The model under review builds one solid part; all positions refer to its coordinate system, in mm. Face numbers are marked on the shaded views. A direction names the side the tool comes from. Coordinates: 2 decimals unless noted, no trailing zeros. Order: outer loops, then holes, each group sorted by start corner. A loop starts at its lowest first (then second) coordinate and runs counter-clockwise, first axis right, second up. Notation, with made-up numbers: (17, 66) - (74, 66) arc R20 ccw to (74, 101) - close; hole circle Ø3 at (-7.75, 13). An arc over 180 degrees is marked (long way). Answer in a Markdown table with one row per item.
Autodesk Inventor part; units mm, degrees
ref_plane "YZ Plane" through (0, 0, 0) normal (1, 0, 0) x (0, 1, 0)
ref_plane "XZ Plane" through (0, 0, 0) normal (0, 1, 0) x (-1, 0, 0)
ref_plane "XY Plane" through (0, 0, 0) normal (0, 0, 1) x (1, 0, 0)
sketch "スケッチ1" plane through (0, 0, 0) normal (1, 0, 0) x (0, 1, 0)
  line L0 (-6.5, 0) -> (6.5, 0)
  line L1 (0, 0) -> (0, 3.1754) construction
  line L2 (-6.2544, 3.1754) -> (-6.5, 2.75)
  line L3 (-6.5, 2.75) -> (-6.5, 0)
  line L4 (-6.2544, 3.1754) -> (6.2544, 3.1754)
  line L5 (6.2544, 3.1754) -> (6.5, 2.75)
  line L6 (6.5, 2.75) -> (6.5, 0)
  line L7 (-6.5, 1.5) -> (-12.2, 1.5)
  line L8 (-12.5, 1.2) -> (-12.5, 0)
  line L9 (-12.5, 0) -> (-6.5, 0)
  line L10 (-12.2, 1.5) -> (-12.5, 1.2)
  point P0 (6.5, 1.5)
  point P1 (-12.5, 1.5)
  dimension "d1" = 2.75
  dimension "d2" = 3.1754
  dimension "d3" = 30
  dimension "d4" = 13
  dimension "d18" = 6
  dimension "d19" = 3
  dimension "d22" = 0.3
  dimension "d23" = 0.3
revolve "回転1" add sketch "スケッチ1" angle 360 about axis through (0, -6.5, 0) along (0, 1, 0)
sketch "スケッチ2" plane through (0, 6.5, 0) normal (0, 1, 0) x (1, 0, 0)
  line L0 (0, -3.1754) -> (-2.75, -1.5877)
  line L1 (-2.75, -1.5877) -> (-2.75, 1.5877)
  line L2 (-2.75, 1.5877) -> (0, 3.1754)
  line L3 (0, 3.1754) -> (2.75, 1.5877)
  line L4 (2.75, 1.5877) -> (2.75, -1.5877)
  line L5 (2.75, -1.5877) -> (0, -3.1754)
  circle A0 centre (0, 0) radius 3.1754
  point P0 (0, 0)
  point P1 (0, 0)
  point P2 (0, 3.1754)
  point P3 (0, 3.1754)
  point P4 (2.75, -1.5877)
  point P5 (2.75, -1.5877)
extrude "押し出し1" cut sketch "スケッチ2" against normal through all contours A0 L0 | L5 A0 | A0 L1 | L4 A0 | A0 L2 | L3 A0
hole "穴1" at (0, 6.5, 0) direction (0, -1, 0) diameter 2.459 depth 3.3 tip angle 118 countersink diameter 3 countersink angle 90
thread "ねじ1"
equation "\"d2\" = 1.1547 * d1"
properties part number "BSL-313BE" material "アセタール樹脂、黒"
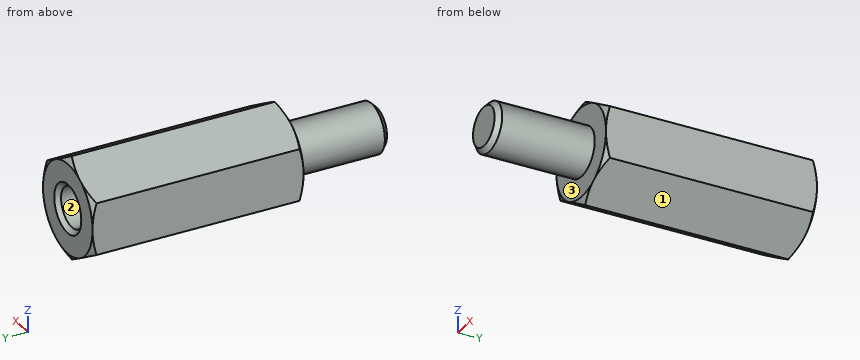
Item 1: We need section A-A, the plane y = 4.25. Write out the cut boundary in (x, z), then the cut area to 3 significant figures.
Check values:
| item | result |
|---|---|
| outline | (-2.75, -1.59) - (0, -3.18) - (2.75, -1.59) - (2.75, 1.59) - (0, 3.18) - (-2.75, 1.59) - close; hole circle Ø2.46 at (0, 0) |
| area | 21.4 mm^2 |
Item 2: Clearance check with a flat-ended pin moving along its axis: pin 1 Ø3 at (x, z) = (1.5, 0.5) entering from -Y. State where the tip first meets the part, or that it passes through.
Check values:
| item | result |
|---|---|
| pin 1 | y = -12.5 |
Item 3: To check wall thickness, follow line 1 (X direction, y = 5, z = 0); line 2 (Y direction, x = 0.9, z = 2); line 3 (Z direction, x = -2.15, y = -3.75). State the ranges of each line that lie inside material, in increasing order. Write a range as from..to.
Check values:
| item | result |
|---|---|
| line 1 | -2.75..-1.23, 1.23..2.75 |
| line 2 | -6.5..6.5 |
| line 3 | -1.93..1.93 |
Item 4: We need section B-B, the plane y = -7. Write out the cut boundary in (x, z).
Check values:
| item | result |
|---|---|
| outline | circle Ø3 at (0, 0) |
Item 5: Tool access review of the marked faces 1, 2 and 3: name each direction out of +Z, -Z, +X, -X, +Y, -Y from which nothing blocks a thin tool from reaching the whole face with its end or side.
Check values:
| item | result |
|---|---|
| face 1 | -Z, +X, +Y, -Y |
| face 2 | +Y |
| face 3 | -Y |
